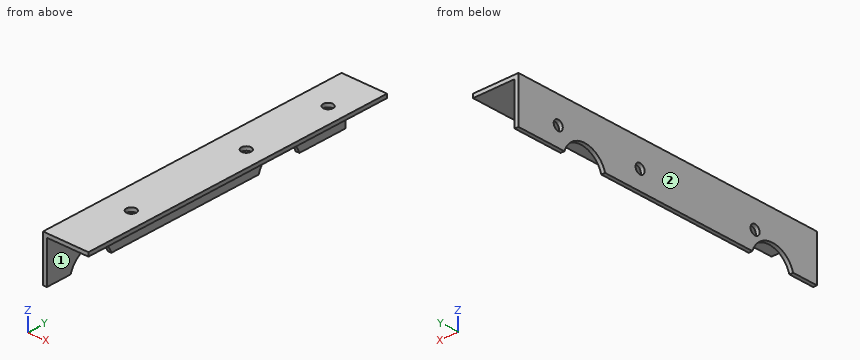
from build123d import *

# Parameters (mm, degrees)
BOSS_EXTRUDE1_DEPTH = 135
SKETCH2_R           = 2.05
CUT_EXTRUDE1_DEPTH  = 138.451232829
SKETCH3_R           = 2.05
CUT_EXTRUDE2_DEPTH  = 138.451232829
SKETCH6_R           = 9.65
CUT_EXTRUDE5_DEPTH  = 10


with BuildPart() as part:
    # Sketch1 → Boss-Extrude1 (new body)
    with BuildSketch(Plane(origin=(0, 0, 0), x_dir=(1, 0, 0), z_dir=(0, 1, 0))):
        Polygon((0, 0), (19.05, 0), (19.05, 1.5875), (1.5875, 1.5875), (1.5875, 19.05), (0, 19.05), align=None)
    extrude(amount=BOSS_EXTRUDE1_DEPTH)

    # Sketch2 → Cut-Extrude1 (cut, through all)
    with BuildSketch(Plane(origin=(1.5875, 0, 0), x_dir=(0, 0, -1), z_dir=(1, 0, 0))):
        with Locations((11.05, 117)):
            Circle(SKETCH2_R)
        with Locations((11.05, 80)):
            Circle(SKETCH2_R)
        with Locations((11.05, 28)):
            Circle(SKETCH2_R)
    extrude(amount=-CUT_EXTRUDE1_DEPTH, mode=Mode.SUBTRACT)

    # Sketch3 → Cut-Extrude2 (cut, through all)
    with BuildSketch(Plane(origin=(0, 0, -1.5875), x_dir=(-1, 0, 0), z_dir=(0, 0, -1))):
        with Locations((-11.05, 117)):
            Circle(SKETCH3_R)
        with Locations((-11.05, 80)):
            Circle(SKETCH3_R)
        with Locations((-11.05, 28)):
            Circle(SKETCH3_R)
    extrude(amount=-CUT_EXTRUDE2_DEPTH, mode=Mode.SUBTRACT)

    # Sketch6 → Cut-Extrude5 (cut)
    with BuildSketch(Plane(origin=(1.5875, 0, 0), x_dir=(0, 0, -1), z_dir=(1, 0, 0))):
        with Locations((21.95, 105)):
            Circle(SKETCH6_R)
        with Locations((21.95, 20)):
            Circle(SKETCH6_R)
    extrude(amount=-CUT_EXTRUDE5_DEPTH, mode=Mode.SUBTRACT)


solid = part.part
Check sheet for the modelled part. Datum: model origin and axes. Units: mm. Face numbers are marked on the shaded views. A direction names the side the tool comes from. Round coordinates to 2 decimals unless told otherwise and drop trailing zeros. Write each loop counter-clockwise with the first axis right and the second up, starting at its lowest first coordinate (ties: lowest second). Pieces come first, ordered by that corner, then holes. Notation, with made-up numbers: (9.5, -2) -> (28.5, -2) arc R19 ccw to (28.5, 24) -> close; hole circle Ø11 at (13.25, -31). An arc over 180 degrees is marked (long way). Answer as CSV lines item,"result". Start each with the question number.
1) Go/stop test with flat-tipped pins: P1, Ø1.5, axis at y = 46.5, z = -11, coming from the +X side; P2, Ø3.5, axis at y = 28, z = -11.05, coming from the +X side; P3, Ø1, axis at x = 4.5, y = 119, coming from the -Z side. Record where each tip stops, or that it passes through.
2) Section check A-A on y = 80. Enter the section's corners in (x, z).
3) Material ranges on line 1 (Y direction, x = 11.05, z = -0.9); line 2 (X direction, y = 123.5, z = -3); line 3 (Z direction, x = 6.5, y = 34), recorded low to high. Write a range as from..to.
4) Section check B-B on z = -11.05. Enter the section's corners in (x, y), and give its area (3 significant figures).
5) Section check C-C on x = 11.05. Enter the section's corners in (y, z), and give its area (3 significant figures).
6) Section check D-D on y = 28. Enter the section's corners in (x, z), and give its area (3 significant figures).
7) Tool access check on the marked faces 1 and 2. Record the directions out of +Z, -Z, +X, -X, +Y, -Y that give a thin tool (end or side, any length) a straight path to the whole face; none if there is none.
Found:
1,P1,"stops at x = 1.59"
1,P2,"passes through"
1,P3,"stops at z = -1.59"
2,outline,"(0, -19.05) -> (1.59, -19.05) -> (1.59, -13.1) -> (0, -13.1) -> close; (0, -9) -> (1.59, -9) -> (1.59, -1.59) -> (9, -1.59) -> (9, 0) -> (0, 0) -> close; (13.1, -1.59) -> (19.05, -1.59) -> (19.05, 0) -> (13.1, 0) -> close"
3,line 1,"y = 0..25.95, 30.05..77.95, 82.05..114.95, 119.05..135"
3,line 2,"x = 0..1.59"
3,line 3,"z = -1.59..0"
4,outline,"(0, 0) -> (1.59, 0) -> (1.59, 25.95) -> (0, 25.95) -> close; (0, 30.05) -> (1.59, 30.05) -> (1.59, 77.95) -> (0, 77.95) -> close; (0, 82.05) -> (1.59, 82.05) -> (1.59, 114.95) -> (0, 114.95) -> close; (0, 119.05) -> (1.59, 119.05) -> (1.59, 135) -> (0, 135) -> close"
4,area,"195 mm^2"
5,outline,"(0, -1.59) -> (25.95, -1.59) -> (25.95, 0) -> (0, 0) -> close; (30.05, -1.59) -> (77.95, -1.59) -> (77.95, 0) -> (30.05, 0) -> close; (82.05, -1.59) -> (114.95, -1.59) -> (114.95, 0) -> (82.05, 0) -> close; (119.05, -1.59) -> (135, -1.59) -> (135, 0) -> (119.05, 0) -> close"
5,area,"195 mm^2"
6,outline,"(0, -16.55) -> (1.59, -16.55) -> (1.59, -13.1) -> (0, -13.1) -> close; (0, -9) -> (1.59, -9) -> (1.59, -1.59) -> (9, -1.59) -> (9, 0) -> (0, 0) -> close; (13.1, -1.59) -> (19.05, -1.59) -> (19.05, 0) -> (13.1, 0) -> close"
6,area,"41.0 mm^2"
7,face 1,"-Z, +X, +Y, -Y"
7,face 2,"+Z, -Z, -X, +Y, -Y"
